```python
from build123d import *

# Parameters (mm, degrees)
F0_R           = 50.8
F1_DEPTH       = 25.4
F3_D           = 6.35
F4_D           = 9.525
F4_CBORE_D     = 19.05
F4_CBORE_DEPTH = 6.35
F5_D           = 9.525
F5_CSINK_D     = 19.05
F5_CSINK_ANGLE = 82
F6_D           = 6.7564
F7_D           = 15.5


with BuildPart() as f1:
    # F0 (on Front) → F1 (new body)
    with BuildSketch(Plane.XZ):
        Circle(F0_R)
    extrude(amount=F1_DEPTH)

    # F3 (through all)
    with Locations(Plane.XZ.offset(25.4)):
        with Locations((30.1960443924, 9.8112895714)):
            Hole(F3_D / 2)

    # F4 (through all)
    with Locations(Plane.XZ.offset(25.4)):
        with Locations((18.6621817603, -25.6862895714)):
            CounterBoreHole(F4_D / 2, F4_CBORE_D / 2, F4_CBORE_DEPTH)

    # F5 (through all)
    with Locations(Plane.XZ.offset(25.4)):
        with Locations((-18.6621817603, -25.6862895714)):
            CounterSinkHole(F5_D / 2, F5_CSINK_D / 2, counter_sink_angle=F5_CSINK_ANGLE)

    # F6 (through all)
    with Locations(Plane.XZ.offset(25.4)):
        with Locations((-30.1960443924, 9.8112895714)):
            Hole(F6_D / 2)

    # F7 (through all)
    with Locations(Plane.XZ.offset(25.4)):
        with Locations((0, 31.75)):
            Hole(F7_D / 2)


solid = f1.part
```
Verification items for the finished model (mm, model axes). A direction names the side the tool comes from. Round coordinates to 2 decimals unless told otherwise and drop trailing zeros. Loops run counter-clockwise (first coordinate to the right, second up) from the corner with the lowest first, then second, coordinate; pieces in that order, holes last. Notation, with made-up numbers: (-20.5, 40.25) -> (6.5, 40.25) arc R34 ccw to (6.5, 72.25) -> close; hole circle Ø7 at (-1, -22). An arc over 180 degrees is marked (long way). Answer as a JSON object with one key per item and string values.
Q1. Section check A-A (x = 0). Record the boundary of the cut face in (y, z).
Data:
{"outline": "(-25.4, -50.8) -> (0, -50.8) -> (0, 24) -> (-25.4, 24) -> close; (-25.4, 39.5) -> (0, 39.5) -> (0, 50.8) -> (-25.4, 50.8) -> close"}
Q2. Section check D-D (z = 21.5). Record the boundary of the cut face in (x, y).
Data:
{"outline": "(-46.03, -25.4) -> (46.03, -25.4) -> (46.03, 0) -> (-46.03, 0) -> close"}
Q3. Section check B-B (z = 36). Record the boundary of the cut face in (x, y), then the cut area to 3 significant figures.
Data:
{"outline": "(-35.84, -25.4) -> (-6.48, -25.4) -> (-6.48, 0) -> (-35.84, 0) -> close; (6.48, -25.4) -> (35.84, -25.4) -> (35.84, 0) -> (6.48, 0) -> close", "area": "1,490 mm2"}
Q4. Scan lines: line 1 (Z direction, x = 0, y = -14.5); line 2 (X direction, y = -14, z = -24); line 3 (X direction, y = -3.25, z = -30). Record each from-to range of solid material in increasing order. Write a range as from..to.
Data:
{"line 1": "z = -50.8..24, 39.5..50.8", "line 2": "x = -44.77..-23.12, -14.21..14.21, 23.12..44.77", "line 3": "x = -41..-20.68, -16.64..16.64, 20.68..41"}
Q5. Go/stop test with flat-tipped pins: P1, Ø1, axis at x = -3, y = -20.5, coming from the -Z side; P2, Ø7.5, axis at x = 18.66, z = -25.69, coming from the +Y side; P3, Ø2, axis at x = 17.5, y = -22.5, coming from the +Z side; P4, Ø6, axis at y = -7, z = 8, coming from the -X side. Record where each tip stops, or that it passes through.
Data:
{"P1": "stops at z = -50.74", "P2": "passes through", "P3": "stops at z = 48.05", "P4": "stops at x = -50.55"}
Q6. Draft check along Z on faces 1 (the flat face through (-1, 0, 1)), 2 (the flat face through (21, -19.05, -21)), 3 (the cylindrical face through (-11.012, -12.522, -49.592)). Enter one of: pulls with the +Z half, pulls with the -Z half, needs draft (parallel to the pull), parting line crosses it, or undercut.
Data:
{"face 1": "needs draft", "face 2": "undercut", "face 3": "parting line crosses it"}
Q7. Section check C-C (y = -13.75). State how many separate pieces and enclosed holes the cut face has, then the cut area to 3 significant figures.
Data:
{"separate pieces": "1", "enclosed holes": "5", "area": "7,710 mm2"}
Q8. Access from +Z, -Z, +X, -X, +Y, -Y to the whole of each face (thin tool, end or side, straight path). Record for faces 4 (the cylindrical face through (16.1, -9.39, -21.67)), 5 (the cylindrical face through (27.461, -22.269, -29.334)).
Data:
{"face 4": "+Y, -Y", "face 5": "-Y"}
